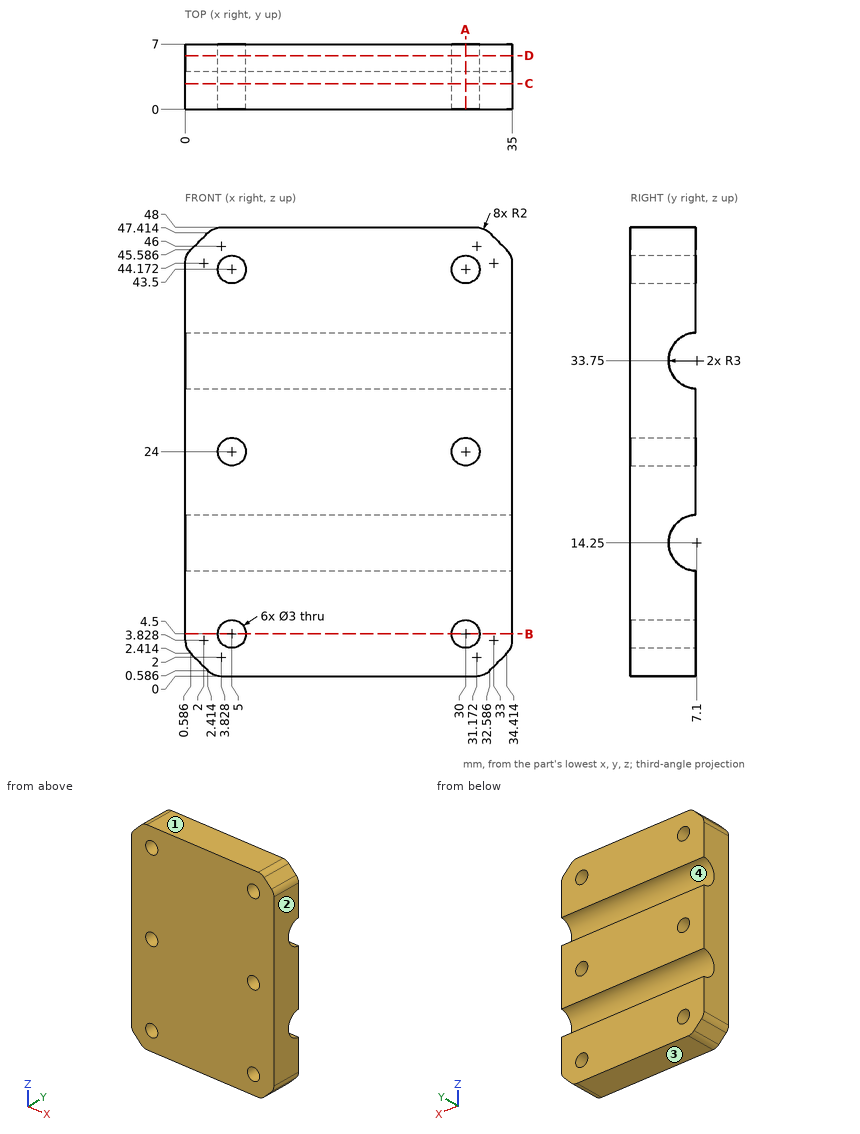
Could you check a few things on this drawing? It's one solid part, dimensions in mm from its lowest x, y, z. Give positions to 0.01 mm unless a question says otherwise; leave off trailing zeros. Write each loop counter-clockwise with the first axis right and the second up, starting at its lowest first coordinate (ties: lowest second). Pieces come first, ordered by that corner, then holes. Notation, with made-up numbers: (77.25, -22.75) -> (121.25, -22.75) arc R31 ccw to (121.25, 3.25) -> close; hole circle Ø8 at (18, 35.5). An arc over 180 degrees is marked (long way). Answer as CSV lines item,"result". Start each with the question number.
(1) If we section it at C-C, the plane y = 2.75: Write out the boundary of the cut face in (x, z) (1 decimal), and give its area (3 significant figures).
(2) If we section it at B-B, the plane z = 4.5: Write out the boundary of the cut face in (x, y), and give its area (3 significant figures).
(3) If we section it at A-A, the plane x = 30: Write out the boundary of the cut face in (y, z).
(4) Please list where these lines run through material, in increasing order: line 1 (X direction, y = 6.25, z = 24); line 2 (Z direction, x = 5, y = 2); line 3 (Z direction, x = 4, y = 0.75).
(5) If we mould it in two halves opening along Z, with no side actions, what happens to the marked faces 1, 2, 3 and 4? For each: +Z half, -Z half, draft (parallel to the pull), parting line (faces both ways), or undercut.
(6) If we section it at D-D, the plane y = 5.75: Give the number of separate pieces and of enclosed holes in the cut face, and give its area (3 significant figures).
(7) I'm going to push a flat-ended pin straight in: pin 1 Ø1.8 at (x, z) = (30, 43.5) entering from -Y. Where does the tip first touch, or does it pass through?
Answer list:
1,outline,"(0, 3.8) arc R2 ccw to (0.6, 2.4) -> (2.4, 0.6) arc R2 ccw to (3.8, 0) -> (31.2, 0) arc R2 ccw to (32.6, 0.6) -> (34.4, 2.4) arc R2 ccw to (35, 3.8) -> (35, 44.2) arc R2 ccw to (34.4, 45.6) -> (32.6, 47.4) arc R2 ccw to (31.2, 48) -> (3.8, 48) arc R2 ccw to (2.4, 47.4) -> (0.6, 45.6) arc R2 ccw to (0, 44.2) -> close; hole circle Ø3 at (5, 4.5); hole circle Ø3 at (5, 24); hole circle Ø3 at (5, 43.5); hole circle Ø3 at (30, 4.5); hole circle Ø3 at (30, 24); hole circle Ø3 at (30, 43.5)"
1,area,"1,620 mm^2"
2,outline,"(0, 0) -> (3.5, 0) -> (3.5, 7) -> (0, 7) -> close; (6.5, 0) -> (28.5, 0) -> (28.5, 7) -> (6.5, 7) -> close; (31.5, 0) -> (35, 0) -> (35, 7) -> (31.5, 7) -> close"
2,area,"203 mm^2"
3,outline,"(0, 0) -> (7, 0) -> (7, 3) -> (0, 3) -> close; (0, 6) -> (7, 6) -> (7, 11.25) arc R3 cw to (7, 17.25) -> (7, 22.5) -> (0, 22.5) -> close; (0, 25.5) -> (7, 25.5) -> (7, 30.75) arc R3 cw to (7, 36.75) -> (7, 42) -> (0, 42) -> close; (0, 45) -> (7, 45) -> (7, 48) -> (0, 48) -> close"
4,line 1,"0 to 3.5, 6.5 to 28.5, 31.5 to 35"
4,line 2,"0 to 3, 6 to 22.5, 25.5 to 42, 45 to 48"
4,line 3,"0 to 3.38, 5.62 to 22.88, 25.12 to 42.38, 44.62 to 48"
5,face 1,"+Z half"
5,face 2,"draft"
5,face 3,"-Z half"
5,face 4,"undercut"
6,separate pieces,"3"
6,enclosed holes,"6"
6,area,"1,240 mm^2"
7,pin 1,"through"
